CAD build for the part. Positions are in the model's coordinates, mm. A direction names the side the tool comes from. Round coordinates to 2 decimals unless told otherwise and drop trailing zeros. Write each loop counter-clockwise with the first axis right and the second up, starting at its lowest first coordinate (ties: lowest second). Pieces come first, ordered by that corner, then holes. Notation, with made-up numbers: (63, -34.75) -> (104, -34.75) arc R33 cw to (104, -5.75) -> close; hole circle Ø10 at (-38.75, 49.5). An arc over 180 degrees is marked (long way). Put each result on its own line as item: value. Start each with the question number.
1. Saw through at D-D on x = -1.5. List the corners of the cut face in (y, z) (3 decimals).
2. Saw through at B-B on x = 0. List the corners of the cut face in (y, z) (3 decimals).
3. Saw through at A-A on z = 0. List the corners of the cut face in (x, y) (3 decimals).
4. 3-axis set-ups, long thin cutter, end or side, ignore diameter. For faces 1 (the cylindrical face through (5.2, 1.1, 0.6)), 2 (the flat face through (1, 0.78, -1)): which of +Z, -Z, +X, -X, +Y, -Y reach the whole face in a straight line?
5. Flat gauge pins, fed straight in: P1, Ø2.5, axis at x = 6, z = 0, coming from the -Y side; P2, Ø4, axis at x = 0, z = 0, coming from the -Y side; P3, Ø2, axis at x = 5, y = 0, coming from the -Z side; P4, Ø2, axis at y = -0.5, z = -1.5, coming from the +X side. Where does each tip first touch, or does it go through?
6. Drill centre lines: line 1 (Z direction, x = 0, y = 1.9); line 2 (X direction, y = 1.3, z = 0); line 3 (Z direction, x = 0, y = 0.2) (3 decimals). Where is each one in solid material? Low to high. Write a range as from..to.
7. Saw through at C-C on y = 0.9. List the corners of the cut face in (x, z).
8. Pull direction Z, two halves, no side cores. Call faces 3 (the cylindrical face through (8.102, 1.06, -2.382)), 4 (the flat face through (4.6, 0, 0)), 5 (the cylindrical face through (-0.471, -0.741, -2.123)), 6 (the cylindrical face through (0.65, 1.47, -1.01)): pulls with the +Z half, pulls with the -Z half, needs draft (parallel to the pull), parting line crosses it, or undercut.
from build123d import *

# Parameters (mm, degrees)
SALIENTE_EXTRUIR1_DEPTH = 2.15
CROQUIS2_R              = 3.5
SALIENTE_EXTRUIR2_DEPTH = 2.22
CROQUIS3_R              = 1.2
CORTAR_EXTRUIR1_DEPTH   = 7.22
CROQUIS4_R              = 2.175
CORTAR_EXTRUIR2_DEPTH   = 3
CROQUIS5_R              = 1
CORTAR_EXTRUIR3_DEPTH   = 10
CUT_EXTRUDE1_DEPTH      = 10
FILLET1_R               = 2


with BuildPart() as part:
    # Croquis1 → Saliente-Extruir1 (new body)
    with BuildSketch(Plane(origin=(0, 0, 0), x_dir=(1, 0, 0), z_dir=(0, 1, 0))):
        with BuildLine():
            Line((0.486006459, 3.466092573), (21.5, 2))
            ThreePointArc((21.5, 2), (23.5, 0), (21.5, -2))
            Line((21.5, -2), (0.486006459, -3.466092573))
            ThreePointArc((0.486006459, -3.466092573), (-3.5, 0), (0.486006459, 3.466092573))
        make_face()
    extrude(amount=SALIENTE_EXTRUIR1_DEPTH)

    # Croquis2 → Saliente-Extruir2 (add)
    with BuildSketch(Plane.XZ):
        Circle(CROQUIS2_R)
    extrude(amount=SALIENTE_EXTRUIR2_DEPTH)

    # Croquis3 → Cortar-Extruir1 (cut)
    with BuildSketch(Plane(origin=(0, 2.15, 0), x_dir=(1, 0, 0), z_dir=(0, 1, 0))):
        Circle(CROQUIS3_R)
    extrude(amount=-CORTAR_EXTRUIR1_DEPTH, mode=Mode.SUBTRACT)

    # Croquis4 → Cortar-Extruir2 (cut)
    with BuildSketch(Plane.XZ.offset(2.22)):
        Circle(CROQUIS4_R)
    extrude(amount=-CORTAR_EXTRUIR2_DEPTH, mode=Mode.SUBTRACT)

    # Croquis5 → Cortar-Extruir3 (cut)
    with BuildSketch(Plane(origin=(0, 2.15, 0), x_dir=(1, 0, 0), z_dir=(0, 1, 0))):
        with Locations((21.5, 0)):
            Circle(CROQUIS5_R)
        with Locations((15.5, 0)):
            Circle(CROQUIS5_R)
        with Locations((6, 0)):
            Circle(CROQUIS5_R)
    extrude(amount=-CORTAR_EXTRUIR3_DEPTH, mode=Mode.SUBTRACT)

    # Sketch1 → Cut-Extrude1 (cut)
    with BuildSketch(Plane(origin=(0, 2.15, 0), x_dir=(1, 0, 0), z_dir=(0, 1, 0))):
        with BuildLine():
            Line((21.5, 2), (8.624907291, 2.898262282))
            Line((8.624907291, 2.898262282), (8.624907291, -2.898262282))
            Line((8.624907291, -2.898262282), (21.5, -2))
            ThreePointArc((21.5, -2), (23.5, 0), (21.5, 2))
        make_face()
    extrude(amount=-CUT_EXTRUDE1_DEPTH, mode=Mode.SUBTRACT)

    # Fillet1
    fillet1_edges = [part.edges().sort_by_distance(p)[0] for p in [
        (8.624907291, 1.075, 2.898262282),
        (8.624907291, 1.075, -2.898262282),
    ]]
    fillet(fillet1_edges, radius=FILLET1_R)


solid = part.part
Return value:
1. outline: (-2.22, -3.162) -> (2.15, -3.162) -> (2.15, 3.162) -> (-2.22, 3.162) -> (-2.22, 1.575) -> (0.78, 1.575) -> (0.78, -1.575) -> (-2.22, -1.575) -> close
2. outline: (-2.22, -3.5) -> (2.15, -3.5) -> (2.15, -1.2) -> (0.78, -1.2) -> (0.78, -2.175) -> (-2.22, -2.175) -> close; (-2.22, 2.175) -> (0.78, 2.175) -> (0.78, 1.2) -> (2.15, 1.2) -> (2.15, 3.5) -> (-2.22, 3.5) -> close
3. outline: (-3.5, -2.22) -> (-2.175, -2.22) -> (-2.175, 0.78) -> (-1.2, 0.78) -> (-1.2, 2.15) -> (-3.5, 2.15) -> close; (1.2, 0.78) -> (2.175, 0.78) -> (2.175, -2.22) -> (3.5, -2.22) -> (3.5, 0) -> (5, 0) -> (5, 2.15) -> (1.2, 2.15) -> close; (7, 0) -> (8.625, 0) -> (8.625, 2.15) -> (7, 2.15) -> close
4. face 1: +Y, -Y
4. face 2: -Y
5. P1: stops at y = 0
5. P2: stops at y = 0.78
5. P3: stops at z = -3.22
5. P4: stops at x = 8.62
6. line 1: z = -3.5..-1.2, 1.2..3.5
6. line 2: x = -3.5..-1.2, 1.2..5, 7..8.62
6. line 3: z = -3.5..-2.175, 2.175..3.5
7. outline: (0.49, -3.47) -> (6.76, -3.03) arc R2 ccw to (8.62, -1.03) -> (8.62, 1.03) arc R2 ccw to (6.76, 3.03) -> (0.49, 3.47) arc R3.5 ccw (long way) to start; hole circle Ø2.4 at (0, 0); hole circle Ø2 at (6, 0)
8. face 3: pulls with the -Z half
8. face 4: needs draft
8. face 5: undercut
8. face 6: undercut
